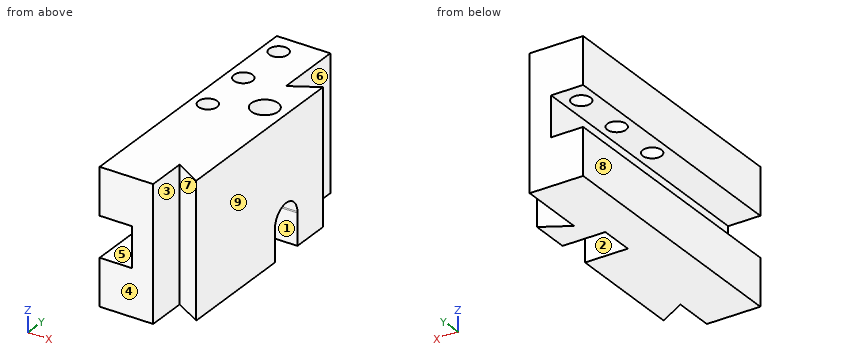
```python
from build123d import *

# Parameters (mm, degrees)
F1_DEPTH = 31.75
F2_W     = 15.24
F2_H     = 9.525
F3_DEPTH = 63.501
F4_R     = 2.2225
F5_DEPTH = 11.1125
F6_R     = 3.175
F7_DEPTH = 25.4
F9_DEPTH = 10.16


# Not quite as in the source:
# - a feature names something its author has since deleted; it is built from what else it names


with BuildPart() as f1:
    # F0 (on Top) → F1 (new body)
    with BuildSketch(Plane.XY):
        Polygon((3.175, 31.75), (-9.525, 31.75), (-9.525, -31.75), (3.175, -31.75), (3.175, -22.225), (3.175, 15.875), align=None)
        Polygon((9.525, 19.5411742094), (3.175, 15.875), (3.175, -22.225), (9.525, -25.8911742094), align=None)
    extrude(amount=F1_DEPTH)

    # F2 (on face) → F3 (cut, through all)
    with BuildSketch(Plane.XZ.offset(31.75)):
        with Locations((-9.525, 15.875)):
            Rectangle(F2_W, F2_H)
    extrude(amount=-F3_DEPTH, mode=Mode.SUBTRACT)

    # F4 (on face) → F5 (cut, through all)
    with BuildSketch(Plane.XY.offset(31.75)):
        with Locations((-5.715, 1.27)):
            Circle(F4_R)
        with Locations((-5.715, 13.97)):
            Circle(F4_R)
        with Locations((-5.715, 26.67)):
            Circle(F4_R)
    extrude(amount=-F5_DEPTH, mode=Mode.SUBTRACT)

    # F6 (on face) → F7 (cut)
    with BuildSketch(Plane.XY.offset(31.75)):
        with Locations((4.445, 6.35)):
            Circle(F6_R)
    extrude(amount=-F7_DEPTH, mode=Mode.SUBTRACT)

    # F8 (on face) → F9 (cut)
    with BuildSketch(Plane.YZ.offset(9.525)):
        with BuildLine():
            Line((10.3787716824, 7.7874478821), (10.3787716824, 7.4525521179))
            ThreePointArc((10.3787716824, 7.4525521179), (10.38225, 7.62), (10.3787716824, 7.7874478821))
        make_face()
        with BuildLine():
            Line((10.3787716824, 0), (10.3787716824, 7.4525521179))
            Line((10.3787716824, 7.4525521179), (10.3787716824, 7.7874478821))
            ThreePointArc((10.3787716824, 7.7874478821), (6.2662579975, 11.6513803268), (2.31775, 7.62))
            Line((2.31775, 7.62), (2.31775, 0))
            Line((2.31775, 0), (10.3787716824, 0))
        make_face()
    extrude(amount=-F9_DEPTH, mode=Mode.SUBTRACT)


solid = f1.part
```
The model under review builds one solid part; all positions refer to its coordinate system, in mm. Face numbers are marked on the shaded views. A direction names the side the tool comes from. Coordinates: 2 decimals unless noted, no trailing zeros. Write each loop counter-clockwise with the first axis right and the second up, starting at its lowest first coordinate (ties: lowest second). Pieces come first, ordered by that corner, then holes. Notation, with made-up numbers: (88.5, 62) -> (125.5, 62) arc R13 ccw to (125.5, 70) -> close; hole circle Ø8 at (45, 65.25). An arc over 180 degrees is marked (long way). One line per item, written item: value. Start each with the question number.
Q1. To check wall thickness, follow probe 1 along X at (y, z) = (6.35, 25.25) (3 decimals); probe 2 along Z at (x, y) = (-4, 5.5); probe 3 along X at (y, z) = (6.35, 14.5) (3 decimals). State the ranges of each line that lie inside material, in increasing order.
Q2. Clearance check with flat-ended pins moving along their axes: P1, Ø3, axis at y = -2, z = 17.5, coming from the -X side (3 decimals); P2, Ø3.5, axis at x = -5.715, y = 1.27, coming from the +Z side; P3, Ø1.5, axis at y = 6.5, z = 10.5, coming from the +X side (3 decimals). State where each tip first meets the part, or that it passes through.
Q3. The part is to be moulded in two halves that separate along Y. For the marked faces 1, 2, 3 and 4, say which applies: +Y half, -Y half, draft (parallel to the pull), parting line (faces both ways), or undercut.
Q4. Add section C-C, the plane z = 24.5. Count the separate pieces of the cut face and the enclosed holes in it, then the cut area to 3 significant figures.
Q5. For the marked faces 5, 6, 7, 8 and 9, list the 3-axis set-ups (+Z, -Z, +X, -X, +Y, -Y) from which the entire face can be reached by the end or side of a thin tool; tool diameter is ignored.
Q6. Add section A-A, the plane x = -2.5. Give the boundary of the cut face in (y, z).
Response:
1. probe 1: -9.525 to 1.27, 7.62 to 9.525
1. probe 2: 0 to 11.11, 20.64 to 31.75
1. probe 3: -1.905 to 1.27, 7.62 to 9.525
2. P1: x = -1.905
2. P2: z = 11.11
2. P3: x = -0.635
3. face 1: undercut
3. face 2: undercut
3. face 3: draft
3. face 4: -Y half
4. separate pieces: 1
4. enclosed holes: 4
4. area: 993 mm²
5. face 5: -X, +Y, -Y
5. face 6: +Z, -Z, +Y
5. face 7: +Z, -Z, -Y
5. face 8: +Z, -Z, -X, +Y, -Y
5. face 9: +Z, -Z, +X, +Y, -Y
6. outline: (-31.75, 0) -> (31.75, 0) -> (31.75, 11.11) -> (-31.75, 11.11) -> close; (-31.75, 20.64) -> (31.75, 20.64) -> (31.75, 31.75) -> (-31.75, 31.75) -> close
